Check sheet for the modelled part. Datum: model origin and axes. Units: mm. A direction names the side the tool comes from. Round coordinates to 2 decimals unless told otherwise and drop trailing zeros. Loops run counter-clockwise (first coordinate to the right, second up) from the corner with the lowest first, then second, coordinate; pieces in that order, holes last. Notation, with made-up numbers: (-10.5, 58.25) -> (3.5, 58.25) arc R31 cw to (3.5, 90.25) -> close; hole circle Ø3 at (77, 53.25). An arc over 180 degrees is marked (long way). One line per item, written item: value. Start each with the question number.
1. Release check for a two-part mould opening along Y. For faces 1 (the face through (0, -20.2, 0)), 2 (the face through (-1, -18, 3)), 3 (the face through (0, 20.2, 0)) record: +Y half, -Y half, draft (parallel to the pull), parting line (faces both ways), or undercut.
2. Material ranges on L1, parallel to Y at x = -2.5, z = -2; L2, parallel to Y at x = -2, z = -2.75; L3, parallel to Z at x = 2.75, y = 2.5, recorded low to high.
3. Cross-section at A-A on y = 16.5. Record the cut outline in (x, z), then the cut area to 3 significant figures.
4. Go/stop test with a flat-tipped pin: pin 1 (3 mm diameter, centred on y = 5.5, z = 2.5, fed in from -X). Record where the tip stops, or that it passes through.
5. Set-up check for faces 4 (the face through (3.417, -19.153, -0.759)), 5 (the face through (-0.9, 18.44, 2.86)): record each of +Z, -Z, +X, -X, +Y, -Y from which the full face is reachable in a straight line by a thin tool's end or side.
from build123d import *


with BuildPart() as part:
    # Esquisse1 → Base-R_volution (revolve)
    with BuildSketch(Plane(origin=(0, 0, 0), x_dir=(-0.25533200274967977, 0, -0.9668534368619877), z_dir=(0.9668534368619877, 0, -0.25533200274967977)), mode=Mode.PRIVATE) as base_r_volution_sk:
        Polygon((-3.5, 18), (-3.5, -18), (-3, -18), (-3, -18.9), (-3.5, -18.9), (-3.5, -19.4), (-2.7, -20.2), (0, -20.2), (0, 20.2), (-2.7, 20.2), (-3.5, 19.4), (-3.5, 18.9), (-3, 18.9), (-3, 18), align=None)
    revolve(base_r_volution_sk.sketch.rotate(Axis((0, 0, 0), (0, -1, 0)), 14.793258758), axis=Axis((0, 0, 0), (0, -1, 0)))


solid = part.part
Taken from the geometry:
1. face 1: -Y half
1. face 2: undercut
1. face 3: +Y half
2. L1: y = -19.7 to -18.9, -18 to 18, 18.9 to 19.7
2. L2: y = -19.5 to -18.9, -18 to 18, 18.9 to 19.5
2. L3: z = -2.17 to 2.17
3. outline: circle Ø7 at (0, 0)
3. area: 38.5 mm2
4. pin 1: stops at x = -3.35
5. face 4: +Y, -Y
5. face 5: none
